Source: three-view drawing plus pictorial views. Frame: mm from the lowest corner of the part. A direction names the side the tool comes from. Give positions to 0.01 mm unless a question says otherwise; leave off trailing zeros. Order: outer loops, then holes, each group sorted by start corner. A loop starts at its lowest first (then second) coordinate and runs counter-clockwise, first axis right, second up. Notation, with made-up numbers: (76, 26) -> (89, 26) arc R21 ccw to (89, 39) -> close; hole circle Ø2 at (6.5, 0.25). An arc over 180 degrees is marked (long way). Use a Markdown table: item, result. Add a question column.
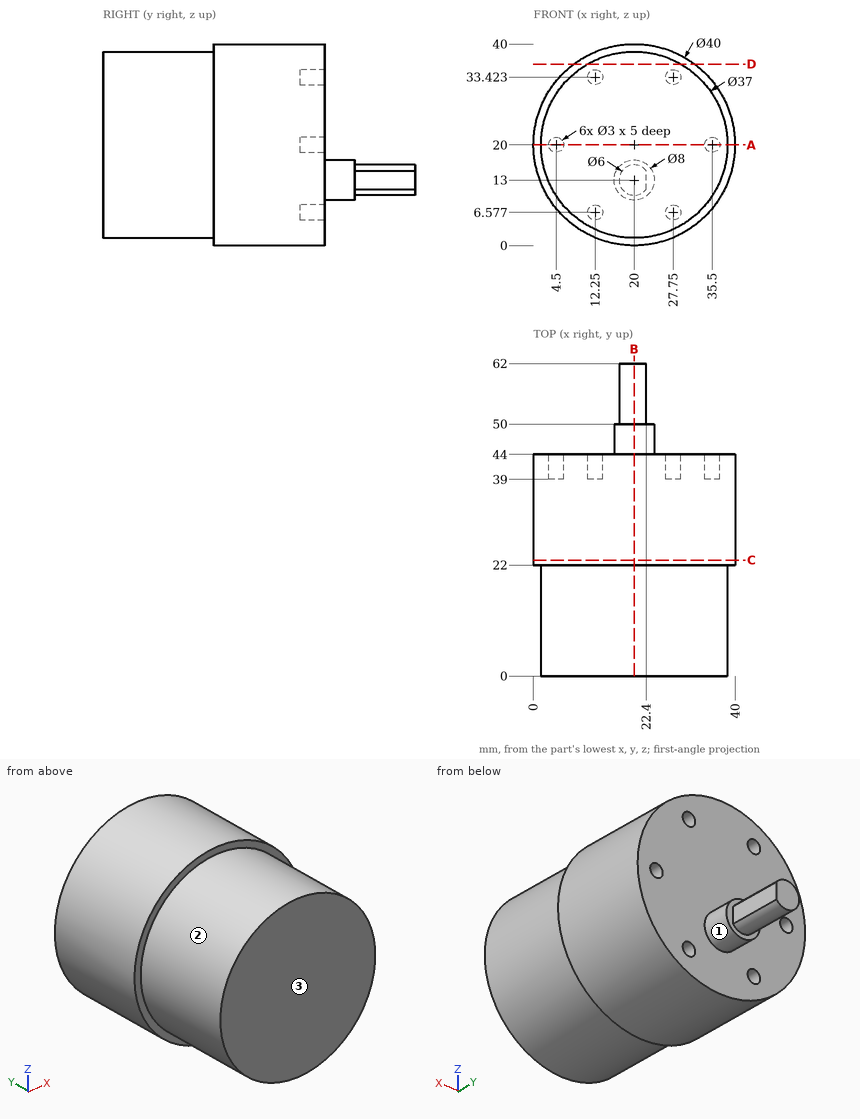
Q1. Access query for the marked faces 1, 2 and 3. Directions: +Z, -Z, +X, -X, +Y, -Y. A direction counts if a zero-diameter tool reaches every point of the face in a straight line with its end or side. Return the directions, or none.
Q2. First-contact query: pin 1 (0.9 mm diameter, centred on x = 28, z = 32.5, fed in from +Y); pin 2 (3.5 mm diameter, centred on x = 12.25, z = 6.58, fed in from +Y); pin 3 (2 mm diameter, centred on y = 9, z = 6.5, fed in from -X); pin 4 (2 mm diameter, centred on x = 11.5, z = 28.5, fed in from -Y). Flat tips, straight axial feed; report the tip coordinate or a pass-through.
Q3. Ray query, line 1 (X direction, y = 40.9, z = 20); line 2 (Z direction, x = 27, y = 41) (1 decimal); line 3 (Y direction, x = 10, z = 12). Return the intervals inside material, ascending.
Q4. Section query A-A (z = 20). Return loops of the section in (x, y).
Q5. Section query D-D (z = 36). Return loops of the section in (x, y), plus the area to 3 significant figures.
Q6. Section query B-B (x = 20). Return loops of the section in (y, z), plus the area to 3 significant figures.
Q7. Section query C-C (y = 23). Return loops of the section in (x, z), plus the area to 3 significant figures.
Solution:
| question | item | result |
|---|---|---|
| 1 | face 1 | +Y |
| 1 | face 2 | -Y |
| 1 | face 3 | +Z, -Z, +X, -X, -Y |
| 2 | pin 1 | stops at y = 39 |
| 2 | pin 2 | stops at y = 44 |
| 2 | pin 3 | stops at x = 6.36 |
| 2 | pin 4 | stops at y = 0 |
| 3 | line 1 | x = 0 to 3, 6 to 34, 37 to 40 |
| 3 | line 2 | z = 1.3 to 5.3, 7.9 to 32.1, 34.7 to 38.7 |
| 3 | line 3 | y = 0 to 44 |
| 4 | outline | (0, 22) -> (1.5, 22) -> (1.5, 0) -> (38.5, 0) -> (38.5, 22) -> (40, 22) -> (40, 44) -> (37, 44) -> (37, 39) -> (34, 39) -> (34, 44) -> (6, 44) -> (6, 39) -> (3, 39) -> (3, 44) -> (0, 44) -> close |
| 5 | outline | (8, 22) -> (10.71, 22) -> (10.71, 0) -> (29.29, 0) -> (29.29, 22) -> (32, 22) -> (32, 44) -> (8, 44) -> close |
| 5 | area | 937 mm² |
| 6 | outline | (0, 1.5) -> (22, 1.5) -> (22, 0) -> (44, 0) -> (44, 9) -> (50, 9) -> (50, 10) -> (62, 10) -> (62, 16) -> (50, 16) -> (50, 17) -> (44, 17) -> (44, 40) -> (22, 40) -> (22, 38.5) -> (0, 38.5) -> close |
| 6 | area | 1,810 mm² |
| 7 | outline | circle Ø40 at (20, 20) |
| 7 | area | 1,260 mm² |
